from build123d import *

# Parameters (mm, degrees)
ESTRUSIONE_ESTRUSIONE1_DEPTH = 5
SCHIZZO2_W                   = 20
SCHIZZO2_H                   = 20
ESTRUSIONE_ESTRUSIONE2_DEPTH = 21
RACCORDO1_RADIUS             = 10
RACCORDO1_LENGTH             = 20
SCHIZZO5_R                   = 6.5
TAGLIO_ESTRUSIONE4_DEPTH     = 57.497787567
SCHIZZO6_R                   = 2.5
TAGLIO_ESTRUSIONE5_DEPTH     = 55.378304497
RACCORDO2_R                  = 6


with BuildPart() as part:
    # Schizzo1 → Estrusione-Estrusione1 (new body)
    with BuildSketch(Plane(origin=(0, 0, 0), x_dir=(1, 0, 0), z_dir=(0, 1, 0))):
        with BuildLine():
            Line((0, 0), (36, 0))
            ThreePointArc((36, 0), (46, -10), (36, -20))
            Line((36, -20), (0, -20))
            ThreePointArc((0, -20), (-10, -10), (0, 0))
        make_face()
    extrude(amount=ESTRUSIONE_ESTRUSIONE1_DEPTH)

    # Schizzo2 → Estrusione-Estrusione2 (add)
    with BuildSketch(Plane(origin=(0, 5, 0), x_dir=(1, 0, 0), z_dir=(0, 1, 0))):
        with Locations((18, -10)):
            Rectangle(SCHIZZO2_W, SCHIZZO2_H)
    extrude(amount=ESTRUSIONE_ESTRUSIONE2_DEPTH)

    # Raccordo1: full round fillet: the end face becomes a half cylinder, R = half its width
    raccordo1_face = Plane((18, 26, 10), x_dir=(0, 0, 1), z_dir=(0, 1, 0))  # on the end face: x along it, z out of the body
    raccordo1_slab = raccordo1_face.offset(-RACCORDO1_RADIUS / 2) * Box(RACCORDO1_LENGTH, 2 * RACCORDO1_RADIUS, RACCORDO1_RADIUS, mode=Mode.PRIVATE)  # the body's end, R deep
    raccordo1_round = Plane((18, 16, 10), x_dir=(0, 1, 0), z_dir=(0, 0, 1)) * Cylinder(RACCORDO1_RADIUS, RACCORDO1_LENGTH, mode=Mode.PRIVATE)  # its axis R under the face
    add(raccordo1_slab - raccordo1_round, mode=Mode.SUBTRACT)

    # Schizzo5 → Taglio-Estrusione4 (cut, through all)
    with BuildSketch(Plane.XY.offset(20)):
        with Locations((18, 16)):
            Circle(SCHIZZO5_R)
    extrude(amount=-TAGLIO_ESTRUSIONE4_DEPTH, mode=Mode.SUBTRACT)

    # Schizzo6 → Taglio-Estrusione5 (cut, through all)
    with BuildSketch(Plane(origin=(0, 5, 0), x_dir=(1, 0, 0), z_dir=(0, 1, 0))):
        with Locations(Location((0, -10, 0), (0, 0, 270))):
            Circle(SCHIZZO6_R)
        with Locations(Location((36, -10, 0), (0, 0, 270))):
            Circle(SCHIZZO6_R)
    extrude(amount=-TAGLIO_ESTRUSIONE5_DEPTH, mode=Mode.SUBTRACT)

    # Raccordo2
    raccordo2_edges = [part.edges().sort_by_distance(p)[0] for p in [
        (8, 5, 10),
        (28, 5, 10),
    ]]
    fillet(raccordo2_edges, radius=RACCORDO2_R)


solid = part.part
Read the model definition and answer for the solid it produces. Units are mm, in the model's axes. A direction names the side the tool comes from. Give positions to 0.01 mm unless a question says otherwise; leave off trailing zeros. Write each loop counter-clockwise with the first axis right and the second up, starting at its lowest first coordinate (ties: lowest second). Pieces come first, ordered by that corner, then holes. Notation, with made-up numbers: (63.5, 42) - (102.5, 42) arc R17 cw to (102.5, 57) - close; hole circle Ø6 at (-28.75, -2.75). An arc over 180 degrees is marked (long way). Use CSV: the item, a comma, the result in double quotes. Start each with the question number.
(1) Given P1, Ø6, axis at x = 36.5, y = 10, coming from the -Z side; P2, Ø1.5, axis at y = 23, z = 9, coming from the -X side; P3, Ø4, axis at y = 14.5, z = 12, coming from the +X side; P4, Ø4, axis at x = 30.5, z = 5.5, coming from the +Y side, each flat-ended and moving along its own axis, determine where each tip first touches the part or whether it passes through.
(2) Find section A-A (x = 18). Give the vertices of the cut face in (y, z), plus the area to 3 significant figures.
(3) Find section B-B (z = 10). Count the separate pieces of the cut face and the enclosed holes in it, plus the area to 3 significant figures.
(4) Consider line 1 along X through (y, z) = (1.75, 10); line 2 along Z through (x, y) = (36, 3.4); line 3 along Y through (x, z) = (18, 11.5). Determine where each line is inside the solid, lowest interval first.
(5) For faces 5 (the cylindrical face through (-10, 2, 10)), 6 (the flat face through (8, 13, 10)), 7 (the flat face through (28, 13, 10)), determine the directions among +Z, -Z, +X, -X, +Y, -Y from which every point of the face is accessible in a straight line to the end or side of a thin tool.
(6) Find section C-C (x = 37). Give the vertices of the cut face in (y, z).
(7) Determine the mould class of faces 1 (the cylindrical face through (46, 2, 10)), 2 (the cylindrical face through (0.1, 2.5, 7.5)), 3 (the flat face through (40, 5, 10)), 4 (the cylindrical face through (33.56, 2.54, 9.46)) for opening direction X: +X half, -X half, draft (parallel to the pull), parting line (faces both ways), or undercut.
Findings below:
1,P1,"through"
1,P2,"x = 10.19"
1,P3,"x = 28"
1,P4,"y = 8.6"
2,outline,"(0, 0) - (9.5, 0) - (9.5, 20) - (0, 20) - close; (22.5, 0) - (26, 0) - (26, 20) - (22.5, 20) - close"
2,area,"260 mm2"
3,separate pieces,"3"
3,enclosed holes,"1"
3,area,"490 mm2"
4,line 1,"-10 to -2.5, 2.5 to 33.5, 38.5 to 46"
4,line 2,"0 to 7.5, 12.5 to 20"
4,line 3,"0 to 9.5, 22.5 to 26"
5,face 5,"-X, +Y, -Y"
5,face 6,"+Z, -Z, -X, +Y"
5,face 7,"+Z, -Z, +X, +Y"
6,outline,"(0, 0.05) - (5, 0.05) - (5, 7.71) - (0, 7.71) - close; (0, 12.29) - (5, 12.29) - (5, 19.95) - (0, 19.95) - close"
7,face 1,"+X half"
7,face 2,"undercut"
7,face 3,"draft"
7,face 4,"undercut"
